Could you check a few things on this model? Use its own coordinates, in mm. A direction names the side the tool comes from. Give positions to 0.01 mm unless a question says otherwise; leave off trailing zeros. Order: outer loops, then holes, each group sorted by start corner. A loop starts at its lowest first (then second) coordinate and runs counter-clockwise, first axis right, second up. Notation, with made-up numbers: (12.25, -19.75) -> (44.25, -19.75) arc R33 ccw to (44.25, 13.25) -> close; hole circle Ø4 at (76.25, 42). An arc over 180 degrees is marked (long way). One line per item, written item: value.
```python
from build123d import *

# Parameters (mm, degrees)
BOSS_EXTRUDE1_DEPTH = 15
BOSS_EXTRUDE2_DEPTH = 60
CUT_EXTRUDE1_DEPTH  = 30
SKETCH4_R           = 6
CUT_EXTRUDE2_DEPTH  = 64
SKETCH5_R           = 7.5
CUT_EXTRUDE3_DEPTH  = 64


with BuildPart() as part:
    # Sketch1 → Boss-Extrude1 (new body)
    with BuildSketch(Plane(origin=(0, 0, 0), x_dir=(1, 0, 0), z_dir=(0, 1, 0))):
        with BuildLine():
            Line((-78, 14.922292207), (-6, 29.619230664))
            ThreePointArc((-6, 29.619230664), (0, 30.22535375), (6, 29.619230664))
            Line((6, 29.619230664), (78, 14.922292207))
            ThreePointArc((78, 14.922292207), (90, 0.22535375), (78, -14.471584706))
            Line((78, -14.471584706), (6, -29.168523163))
            ThreePointArc((6, -29.168523163), (0, -29.77464625), (-6, -29.168523163))
            Line((-6, -29.168523163), (-78, -14.471584706))
            ThreePointArc((-78, -14.471584706), (-90, 0.22535375), (-78, 14.922292207))
        make_face()
    extrude(amount=BOSS_EXTRUDE1_DEPTH)

    # Sketch2 → Boss-Extrude2 (add)
    with BuildSketch(Plane(origin=(0, 15, 0), x_dir=(1, 0, 0), z_dir=(0, 1, 0))):
        with BuildLine():
            Line((-29.023299464, 7.5), (29.023299464, 7.5))
            ThreePointArc((29.023299464, 7.5), (0, 29.976689473), (-29.023299464, 7.5))
        make_face()
        with BuildLine():
            Line((-29.023299464, -7.5), (29.023299464, -7.5))
            ThreePointArc((29.023299464, -7.5), (0, -29.976689473), (-29.023299464, -7.5))
        make_face()
    extrude(amount=BOSS_EXTRUDE2_DEPTH)

    # Sketch3 → Cut-Extrude1 (cut)
    with BuildSketch(Plane(origin=(0, 75, 0), x_dir=(1, 0, 0), z_dir=(0, 1, 0))):
        with BuildLine():
            Line((-24.366985862, 17.5), (24.366985862, 17.5))
            ThreePointArc((24.366985862, 17.5), (0, 30), (-24.366985862, 17.5))
        make_face()
        with BuildLine():
            Line((-24.366985862, -17.5), (24.366985862, -17.5))
            ThreePointArc((24.366985862, -17.5), (0, -30), (-24.366985862, -17.5))
        make_face()
    extrude(amount=-CUT_EXTRUDE1_DEPTH, mode=Mode.SUBTRACT)

    # Sketch4 → Cut-Extrude2 (cut)
    with BuildSketch(Plane.XY.offset(17.5)):
        with Locations((0, 60)):
            Circle(SKETCH4_R)
    extrude(amount=-CUT_EXTRUDE2_DEPTH, mode=Mode.SUBTRACT)

    # Sketch5 → Cut-Extrude3 (cut)
    with BuildSketch(Plane(origin=(0, 15, 0), x_dir=(1, 0, 0), z_dir=(0, 1, 0))):
        with Locations(Location((-75, 0.22535375, 0), (0, 0, 270))):
            Circle(SKETCH5_R)
        with Locations(Location((75, 0.22535375, 0), (0, 0, 270))):
            Circle(SKETCH5_R)
    extrude(amount=-CUT_EXTRUDE3_DEPTH, mode=Mode.SUBTRACT)


solid = part.part
```
1) For faces 4 (the flat face through (0, 45, -22)), 5 (the cylindrical face through (0.085, 7.395, 29.775)), 6 (the flat face through (1, 15, -1)), 7 (the flat face through (-6, 64, 17.5)), which set-ups out of +Z, -Z, +X, -X, +Y, -Y let a thin tool reach every point of the face, with its end or its side?
Answer below:
face 4: -Z, +X, -X, +Y
face 5: +Z, -Y
face 6: +Y
face 7: +Z, +X, -X, +Y
2) Suppose I cut it at A-A, the plane x = 0. Write out the boundary of the cut face in (y, z).
Answer below:
outline: (0, -30.23) -> (15, -30.23) -> (15, -29.98) -> (45, -29.98) -> (45, -17.5) -> (54, -17.5) -> (54, -7.5) -> (15, -7.5) -> (15, 7.5) -> (54, 7.5) -> (54, 17.5) -> (45, 17.5) -> (45, 29.98) -> (15, 29.98) -> (15, 29.77) -> (0, 29.77) -> close; (66, -17.5) -> (75, -17.5) -> (75, -7.5) -> (66, -7.5) -> close; (66, 7.5) -> (75, 7.5) -> (75, 17.5) -> (66, 17.5) -> close
3) Suppose I cut it at C-C, the plane z = 2.5. Write out the boundary of the cut face in (x, y).
Answer below:
outline: (-89.75, 0) -> (-81.99, 0) -> (-81.99, 15) -> (-89.75, 15) -> close; (-68.01, 0) -> (68.01, 0) -> (68.01, 15) -> (-68.01, 15) -> close; (81.99, 0) -> (89.75, 0) -> (89.75, 15) -> (81.99, 15) -> close
4) We'd pull the mould along Y, two halves only. Please class faces 1 (the cylindrical face through (-4.42, 64.06, -12.43)), 2 (the flat face through (0, 45, 22)), 3 (the flat face through (-42.5, 7.4, -22.17)): +Y half, -Y half, draft (parallel to the pull), parting line (faces both ways), or undercut.
Answer below:
face 1: undercut
face 2: +Y half
face 3: draft
5) If I drill on line 1 along X through (y, z) = (12, 5.5); line 2 along Y through (x, z) = (0, 15); line 3 along Z through (x, y) = (1.5, 21.5), over which ranges is the centre line in solid material (lowest first)?
Answer below:
line 1: x = -88.86 to -79.84, -70.16 to 70.16, 79.84 to 88.86
line 2: y = 0 to 54, 66 to 75
line 3: z = -29.94 to -7.5, 7.5 to 29.94
6) For P1, Ø8, axis at x = -4.5, z = -6.5, coming from the +Y side; P2, Ø24, axis at x = 9, y = 62.5, coming from the +Z side; P3, Ø1.5, axis at y = 14.5, z = 12, coming from the +X side; P4, Ø12, axis at x = 21, y = 62, coming from the -Z side, each with a flat end and sliding along its axis, tell me the tip position at first contact or that it passes through.
Answer below:
P1: stops at y = 75
P2: stops at z = 17.5
P3: stops at x = 84.66
P4: stops at z = -17.5
7) Suppose I cut it at D-D, the plane x = 75. Write out the boundary of the cut face in (y, z).
Answer below:
outline: (0, -15.53) -> (15, -15.53) -> (15, -7.73) -> (0, -7.73) -> close; (0, 7.27) -> (15, 7.27) -> (15, 15.08) -> (0, 15.08) -> close
8) Suppose I cut it at B-B, the plane y = 26.5. Write out the boundary of the cut face in (x, z), then the cut area to 3 significant figures.
Answer below:
outline: (-29.02, -7.5) arc R29.98 ccw to (29.02, -7.5) -> close; (-29.02, 7.5) -> (29.02, 7.5) arc R29.98 ccw to start
area: 1,930 mm2
